Part print with two shaded views. Sizes in mm from the minimum x, y, z corner. A direction names the side the tool comes from. Round coordinates to 2 decimals unless told otherwise and drop trailing zeros. Write each loop counter-clockwise with the first axis right and the second up, starting at its lowest first coordinate (ties: lowest second). Pieces come first, ordered by that corner, then holes. Notation, with made-up numbers: (-27.75, 71.5) - (15.25, 71.5) arc R25 ccw to (15.25, 89.5) - close; hole circle Ø3 at (58, -13). An arc over 180 degrees is marked (long way). Answer as a JSON object with one key per item and string values. Group by question number.
Item 1: Slice it at A-A, the plane y = 30. List the corners of the cut face in (x, z).
Item 2: Slice it at B-B, the plane x = 110. List the corners of the cut face in (y, z), then the cut area to 3 significant figures.
Item 3: Slice it at D-D, the plane x = 227. List the corners of the cut face in (y, z), then the cut area to 3 significant figures.
Item 4: Slice it at C-C, the plane z = 22.25. List the corners of the cut face in (x, y).
Item 5: Flat gauge pins, fed straight in: pin 1 (10 mm diameter, centred on x = 63.5, y = 8.5, fed in from +Z); pin 2 (4.5 mm diameter, centred on x = 110, y = 30, fed in from +Z). Where does each tip first touch, or does it go through?
Item 6: Probe line 1 (Y direction, x = 219, z = 10.75); line 2 (Y direction, x = 110, z = 1.3); line 3 (Z direction, x = 111, y = 5). List the from-to ranges inside material, lowest first. Write a range as from..to.
Item 7: Which spindle directions (+Z, -Z, +X, -X, +Y, -Y) get a long thin tool onto all of the face, cutting with end or side? Do the marked faces 1 and 2. Say none if no direction does.
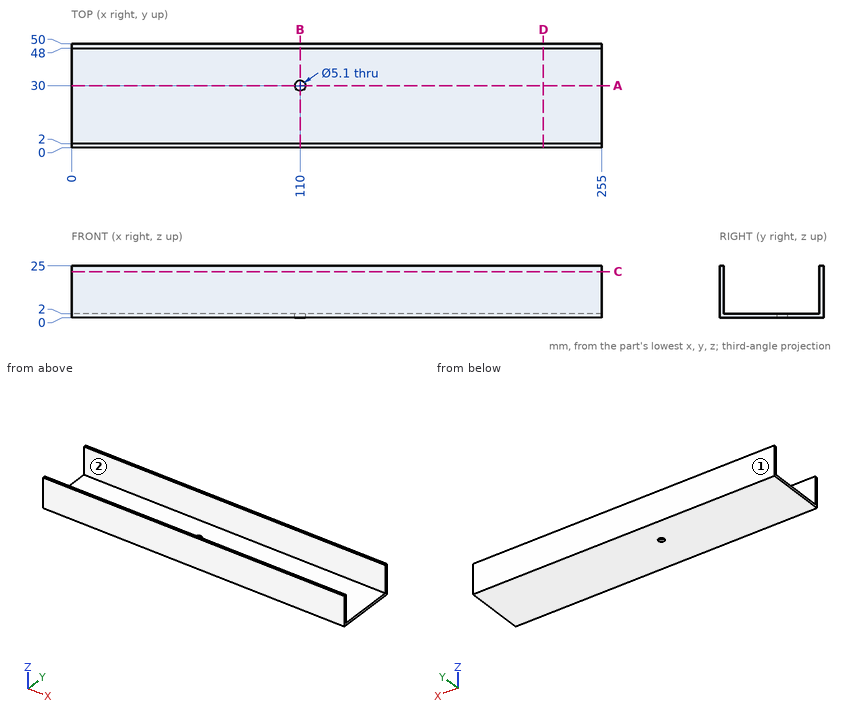
Geometry says:
{
 "1": {"outline": "(0, 0) - (107.45, 0) - (107.45, 2) - (0, 2) - close; (112.55, 0) - (255, 0) - (255, 2) - (112.55, 2) - close"},
 "2": {"outline": "(0, 0) - (27.45, 0) - (27.45, 2) - (2, 2) - (2, 25) - (0, 25) - close; (32.55, 0) - (50, 0) - (50, 25) - (48, 25) - (48, 2) - (32.55, 2) - close", "area": "182 mm^2"},
 "3": {"outline": "(0, 0) - (50, 0) - (50, 25) - (48, 25) - (48, 2) - (2, 2) - (2, 25) - (0, 25) - close", "area": "192 mm^2"},
 "4": {"outline": "(0, 0) - (255, 0) - (255, 2) - (0, 2) - close; (0, 48) - (255, 48) - (255, 50) - (0, 50) - close"},
 "5": {"pin 1": "stops at z = 2", "pin 2": "passes through"},
 "6": {"line 1": "y = 0..2, 48..50", "line 2": "y = 0..27.45, 32.55..50", "line 3": "z = 0..2"},
 "7": {"face 1": "+Z, -Z, +X, -X, +Y", "face 2": "+Z, +X, -X"}
}
